The listing builds one solid part. Answer for the finished solid, in the listing's coordinates (mm). A direction names the side the tool comes from. Give positions to 0.01 mm unless a question says otherwise; leave off trailing zeros. Loops run counter-clockwise (first coordinate to the right, second up) from the corner with the lowest first, then second, coordinate; pieces in that order, holes last. Notation, with made-up numbers: (-32, 86.5) - (-3, 86.5) arc R12 ccw to (-3, 100.5) - close; hole circle Ø5 at (-26.75, 76). An arc over 180 degrees is marked (long way). Answer as CSV lines item,"result". Start each with the question number.
1) For a pull along Y with two mould halves and no side action, classify faces 1 (the face through (1, 0, 9)), 2 (the face through (-51, 12, 23)), 3 (the face through (1, 21.83, 11)) as pulls with the +Y half, pulls with the -Y half, needs draft (parallel to the pull), parting line crosses it, or undercut.
2) Find the intervals of material crossed by line 1 along Y through (x, z) = (14.5, 6.25); line 2 along Y through (x, z) = (17, 21); line 3 along Z through (x, y) = (-18.5, 7.25), in increasing order.
3) A cutting plane is placed at A-A (z = 16.25). Determine the outline of the cut face in (x, y), and give its area (3 significant figures).
4) A cutting plane is placed at D-D (y = 20.25). Determine the outline of the cut face in (x, z), and give its area (3 significant figures).
5) Flat-ended cylindrical pins translate along their axes: pin 1 (3 mm diameter, centred on x = -30.5, z = 22, fed in from -Y); pin 2 (1 mm diameter, centred on x = -17.5, y = 5, fed in from +Z). Find the tip coordinate at first contact, or state that the pin passes through.
6) A cutting plane is placed at B-B (x = -13). Determine the outline of the cut face in (y, z), and give its area (3 significant figures).
7) A cutting plane is placed at C-C (y = 16). Determine the outline of the cut face in (x, z), and give its area (3 significant figures).
8) For faces 4 (the face through (1, 25, 9)), 5 (the face through (1, 3.17, 11)), determine the directions among +Z, -Z, +X, -X, +Y, -Y from which every point of the face is accessible in a straight line to the end or side of a thin tool.
```python
from build123d import *

# Parameters (mm, degrees)
F1_DEPTH = 51
F2_R     = 6.35


with BuildPart() as f1:
    # F0 (on Right) → F1 (new body, symmetric)
    with BuildSketch(Plane.YZ):
        Polygon((0, 25), (0, 0), (3.17, 0), (3.17, 21.83), (21.83, 21.83), (21.83, 0), (25, 0), (25, 25), align=None)
    extrude(amount=F1_DEPTH, both=True)

    # F2
    f2_edges = [f1.edges().sort_by_distance(p)[0] for p in [
        (0, 25, 25),
        (0, 0, 25),
    ]]
    fillet(f2_edges, radius=F2_R)


solid = f1.part
```
Ans:
1,face 1,"pulls with the -Y half"
1,face 2,"needs draft"
1,face 3,"undercut"
2,line 1,"0 to 3.17, 21.83 to 25"
2,line 2,"0.45 to 3.17, 21.83 to 24.55"
2,line 3,"21.83 to 25"
3,outline,"(-51, 0) - (51, 0) - (51, 3.17) - (-51, 3.17) - close; (-51, 21.83) - (51, 21.83) - (51, 25) - (-51, 25) - close"
3,area,"647 mm2"
4,outline,"(-51, 21.83) - (51, 21.83) - (51, 24.8) - (-51, 24.8) - close"
4,area,"302 mm2"
5,pin 1,"y = 0.28"
5,pin 2,"z = 24.94"
6,outline,"(0, 0) - (3.17, 0) - (3.17, 21.83) - (21.83, 21.83) - (21.83, 0) - (25, 0) - (25, 18.65) arc R6.35 ccw to (18.65, 25) - (6.35, 25) arc R6.35 ccw to (0, 18.65) - close"
6,area,"200 mm2"
7,outline,"(-51, 21.83) - (51, 21.83) - (51, 25) - (-51, 25) - close"
7,area,"323 mm2"
8,face 4,"+Z, -Z, +X, -X, +Y"
8,face 5,"-Z, +X, -X"
